Verification items for this drawing (mm, ordinates from the low corner). A direction names the side the tool comes from. Round coordinates to 2 decimals unless told otherwise and drop trailing zeros. Loops run counter-clockwise (first coordinate to the right, second up) from the corner with the lowest first, then second, coordinate; pieces in that order, holes last. Notation, with made-up numbers: (-14, 46.5) - (27, 46.5) arc R20 cw to (27, 68.5) - close; hole circle Ø7 at (-9, -2). An arc over 180 degrees is marked (long way). Answer in a Markdown table with one row per item. Add a question column.
(1) Cross-section at C-C on y = 0.55. Enter the section's corners in (x, z).
(2) Cross-section at B-B on z = 6. Enter the section's corners in (x, y), then the cut area to 3 significant figures.
(3) Mould release check, pull along Z, two halves, no side actions. Record for the marked faces 1, 2 and 3: +Z half, -Z half, draft (parallel to the pull), parting line (faces both ways), or undercut.
(4) Cross-section at A-A on x = 6. Enter the section's corners in (y, z), then the cut area to 3 significant figures.
(5) Access from +Z, -Z, +X, -X, +Y, -Y to the whole of each face (thin tool, end or side, straight path). Record for the marked faces 4 and 5.
(6) Gauge pin test, flat end, axial feed: pin 1 (1 mm diameter, centred on x = 10.5, z = 3, fed in from +Y). Record the tip position at first contact, or that the pin passes through.
(7) Cross-section at D-D on y = 2.5. Enter the section's corners in (x, z).
(8) Thickness scan on line 1 along Z through (x, y) = (6, 2.2); line 2 along Z through (x, y) = (6, 1.6); line 3 along X through (y, z) = (2.3, 7.5). Record the ranges inside material, lowest first.
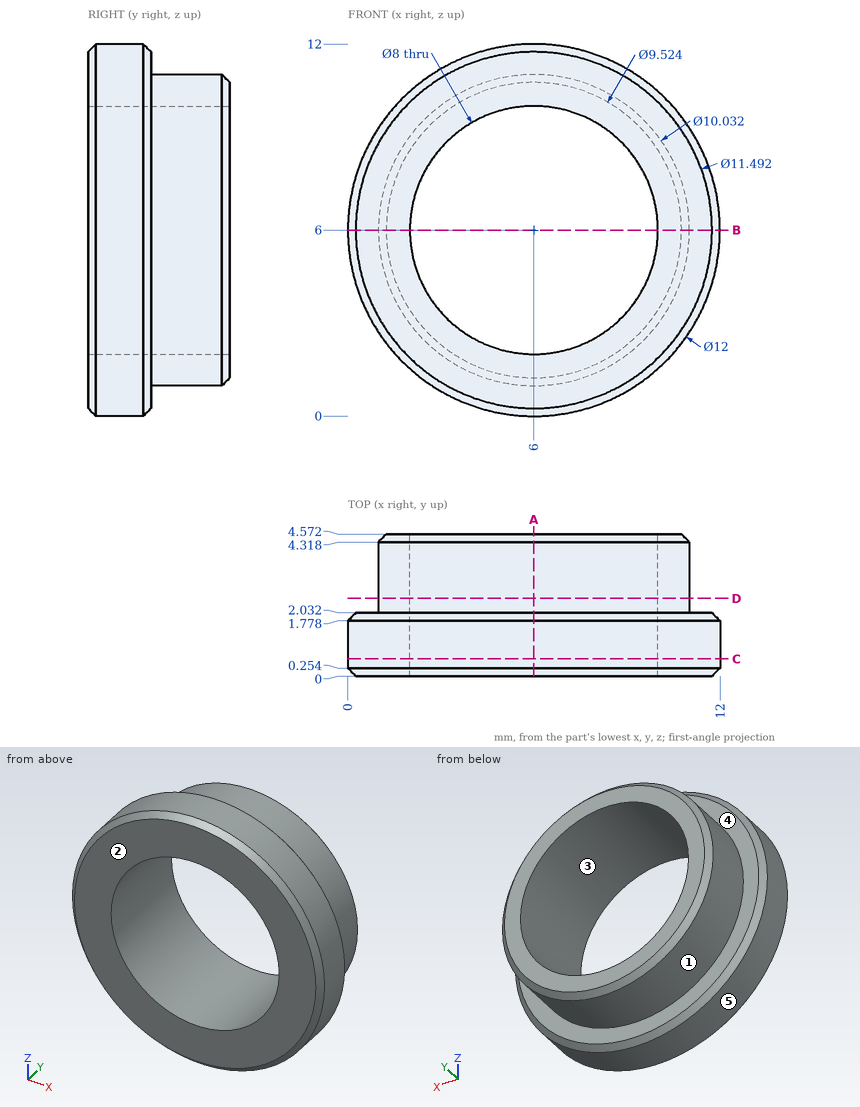
Answers:
| question | item | result |
|---|---|---|
| 1 | outline | circle Ø12 at (6, 6); hole circle Ø8 at (6, 6) |
| 2 | outline | (0, 0.25) - (0.25, 0) - (2, 0) - (2, 4.57) - (1.24, 4.57) - (0.98, 4.32) - (0.98, 2.03) - (0.25, 2.03) - (0, 1.78) - close; (10, 0) - (11.75, 0) - (12, 0.25) - (12, 1.78) - (11.75, 2.03) - (11.02, 2.03) - (11.02, 4.32) - (10.76, 4.57) - (10, 4.57) - close |
| 2 | area | 13.1 mm^2 |
| 3 | face 1 | parting line |
| 3 | face 2 | draft |
| 3 | face 3 | undercut |
| 4 | outline | (0, 0.25) - (0.25, 0) - (1.78, 0) - (2.03, 0.25) - (2.03, 0.98) - (4.32, 0.98) - (4.57, 1.24) - (4.57, 2) - (0, 2) - close; (0, 10) - (4.57, 10) - (4.57, 10.76) - (4.32, 11.02) - (2.03, 11.02) - (2.03, 11.75) - (1.78, 12) - (0.25, 12) - (0, 11.75) - close |
| 4 | area | 13.1 mm^2 |
| 5 | face 4 | +Y |
| 5 | face 5 | +Y, -Y |
| 6 | pin 1 | stops at y = 4.43 |
| 7 | outline | circle Ø10.03 at (6, 6); hole circle Ø8 at (6, 6) |
| 8 | line 1 | z = 0.98 to 2, 10 to 11.02 |
| 8 | line 2 | z = 0 to 2, 10 to 12 |
| 8 | line 3 | x = 1.21 to 2.29, 9.71 to 10.79 |
